from build123d import *

# Parameters (mm, degrees)
EXTRUDE_1_DEPTH     = 6.5
CUT_EXTRUDE_1_REACH = 7
SKETCH_3_R          = 1
CUT_EXTRUDE_2_DEPTH = 3.5
CUT_EXTRUDE_3_DEPTH = 0.5
FILLET_1_R          = 0.2


with BuildPart() as part:
    # 草图1 → 凸台-拉伸1 (new body)
    with BuildSketch(Plane(origin=(0, 0, 0), x_dir=(1, 0, 0), z_dir=(0, 1, 0))):
        with BuildLine():
            Line((-19, 2.5), (19, 2.5))
            ThreePointArc((19, 2.5), (21.5, 0), (19, -2.5))
            Line((19, -2.5), (-19, -2.5))
            ThreePointArc((-19, -2.5), (-21.5, 0), (-19, 2.5))
        make_face()
    extrude(amount=EXTRUDE_1_DEPTH)

    # 草图2 → 切除-拉伸1 (cut, up to next)
    with BuildSketch(Plane.XY.offset(2.5), mode=Mode.PRIVATE) as cut_extrude_1_sk1:
        Polygon((17.468871126, 6.5), (21.5, 4.5), (21.5, 7.438332244), (17.468871126, 7.438332244), align=None)
    cut_extrude_1_tool1 = extrude(cut_extrude_1_sk1.sketch, amount=-CUT_EXTRUDE_1_REACH, mode=Mode.PRIVATE) & part.part
    add(cut_extrude_1_tool1.solids().sort_by_distance((19.83105, 6.383182, 2.5))[0], mode=Mode.SUBTRACT)
    # 草图2 → 切除-拉伸1 (cut, up to next)
    with BuildSketch(Plane.XY.offset(2.5), mode=Mode.PRIVATE) as cut_extrude_1_sk2:
        Polygon((14, 4), (16.5, 0), (16.5, -3.02965668), (-16.5, -3.02965668), (-16.5, 0), (-14, 4), align=None)
    cut_extrude_1_tool2 = extrude(cut_extrude_1_sk2.sketch, amount=-CUT_EXTRUDE_1_REACH, mode=Mode.PRIVATE) & part.part
    add(cut_extrude_1_tool2.solids().sort_by_distance((0, 0.386897, 2.5))[0], mode=Mode.SUBTRACT)
    # 草图2 → 切除-拉伸1 (cut, up to next)
    with BuildSketch(Plane.XY.offset(2.5), mode=Mode.PRIVATE) as cut_extrude_1_sk3:
        Polygon((-21.5, 7.438332244), (-17.468871126, 7.438332244), (-17.468871126, 6.5), (-21.5, 4.5), align=None)
    cut_extrude_1_tool3 = extrude(cut_extrude_1_sk3.sketch, amount=-CUT_EXTRUDE_1_REACH, mode=Mode.PRIVATE) & part.part
    add(cut_extrude_1_tool3.solids().sort_by_distance((-19.83105, 6.383182, 2.5))[0], mode=Mode.SUBTRACT)

    # 草图3 → 切除-拉伸2 (cut)
    with BuildSketch(Plane.XZ):
        with Locations((18.75, 0)):
            Circle(SKETCH_3_R)
        with Locations((-18.75, 0)):
            Circle(SKETCH_3_R)
    extrude(amount=-CUT_EXTRUDE_2_DEPTH, mode=Mode.SUBTRACT)

    # 草图4 → 切除-拉伸3 (cut)
    with BuildSketch(Plane(origin=(0, 6.5, 0), x_dir=(1, 0, 0), z_dir=(0, 1, 0))):
        with BuildLine():
            Line((-9, 1), (9, 1))
            ThreePointArc((9, 1), (10, 0), (9, -1))
            Line((9, -1), (-9, -1))
            ThreePointArc((-9, -1), (-10, 0), (-9, 1))
        make_face()
    extrude(amount=-CUT_EXTRUDE_3_DEPTH, mode=Mode.SUBTRACT)

    # 圆角1
    fillet_1_edges = [part.edges().sort_by_distance(p)[0] for p in [
        (-10, 6, 0),
        (0, 6, -1),
        (10, 6, 0),
        (0, 6, 1),
    ]]
    fillet(fillet_1_edges, radius=FILLET_1_R)


solid = part.part
Geometry: final body of the model. Coordinates: model frame, mm. A direction names the side the tool comes from. Give positions to 0.01 mm unless a question says otherwise; leave off trailing zeros. Write each loop counter-clockwise with the first axis right and the second up, starting at its lowest first coordinate (ties: lowest second). Pieces come first, ordered by that corner, then holes. Notation, with made-up numbers: M 46.25,38 L 69.25,38 A19 ccw 69.25,65 Z; hole C -34.5,5 d11. An arc over 180 degrees is marked long. Answer in a Markdown table with one row per item. Add a question column.
(1) First-contact query: pin 1 (1.5 mm diameter, centred on y = 2, z = 2, fed in from +X); pin 2 (1.5 mm diameter, centred on x = -4.5, y = 1.5, fed in from +Z); pin 3 (0.5 mm diameter, centred on x = -2, z = 0.5, fed in from +Y); pin 4 (2.5 mm diameter, centred on x = 4, z = -0.5, fed in from -Y). Flat tips, straight axial feed; report the tip coordinate or a pass-through.
(2) Ray query, line 1 (Z direction, x = -18.75, y = 2.4); line 2 (X direction, y = 2.25, z = -0.7); line 3 (X direction, y = 2.75, z = 0.25). Return the intervals inside material, ascending.
(3) Section D-D on y = 5. Return loops of the section in (x, z).
(4) Reachability of faces 1 (the flat face through (15.23, 2.03, 0.04)), 2 (the flat face through (0, 6, 0)), 3 (the flat face through (-19, 3.5, 0)) from +Z, -Z, +X, -X, +Y, -Y: full face, straight path, thin tool, end or side. Return the list, or none.
(5) Section C-C on z = 0. Return loops of the section in (x, y), and give its area (3 significant figures).
(6) Section B-B on x = -4. Return loops of the section in (y, z), and give its area (3 significant figures).
(7) Section A-A on y = 2. Return loops of the section in (x, z), and give its area (3 significant figures).
(8) Mould query, pull axis X, two halves, no side actions, for faces 4 (the flat face through (-15.27, 1.97, 0.04)), 5 (the cylindrical face through (21.5, 2.2, -0.1)), 6 (the cylindrical face through (-21.5, 2.2, 0.1)), 7 (the flat face through (0, 4, 0)). Classes: +X half, -X half, draft (parallel to the pull), parting line (faces both ways), or undercut.
Result set:
| question | item | result |
|---|---|---|
| 1 | pin 1 | stops at x = 21.17 |
| 1 | pin 2 | passes through |
| 1 | pin 3 | stops at y = 6 |
| 1 | pin 4 | stops at y = 4 |
| 2 | line 1 | z = -2.5 to -1, 1 to 2.5 |
| 2 | line 2 | x = -21.4 to -19.46, -18.04 to -15.09, 15.09 to 18.04, 19.46 to 21.4 |
| 2 | line 3 | x = -21.49 to -19.72, -17.78 to -14.78, 14.78 to 17.78, 19.72 to 21.49 |
| 3 | outline | M -20.49,-2.01 A2.5 ccw -19,-2.5 L 19,-2.5 A2.5 ccw 20.49,-2.01 L 20.49,2.01 A2.5 ccw 19,2.5 L -19,2.5 A2.5 ccw -20.49,2.01 Z |
| 4 | face 1 | +Z, -Z, -Y |
| 4 | face 2 | +Y |
| 4 | face 3 | -Y |
| 5 | outline | M -21.5,0 L -19.75,0 L -19.75,3.5 L -17.75,3.5 L -17.75,0 L -16.5,0 L -14,4 L 14,4 L 16.5,0 L 17.75,0 L 17.75,3.5 L 19.75,3.5 L 19.75,0 L 21.5,0 L 21.5,4.5 L 17.47,6.5 L 10,6.5 L 10,6.2 A0.2 cw 9.8,6 L -9.8,6 A0.2 cw -10,6.2 L -10,6.5 L -17.47,6.5 L -21.5,4.5 Z |
| 5 | area | 125 mm^2 |
| 6 | outline | M 4,-2.5 L 6.5,-2.5 L 6.5,-1 L 6.2,-1 A0.2 cw 6,-0.8 L 6,0.8 A0.2 cw 6.2,1 L 6.5,1 L 6.5,2.5 L 4,2.5 Z |
| 6 | area | 11.5 mm^2 |
| 7 | outline | M -19,-2.5 L -15.25,-2.5 L -15.25,2.5 L -19,2.5 A2.5 ccw Z; M 15.25,-2.5 L 19,-2.5 A2.5 ccw 19,2.5 L 15.25,2.5 Z; hole C -18.75,0 d2; hole C 18.75,0 d2 |
| 7 | area | 50.9 mm^2 |
| 8 | face 4 | undercut |
| 8 | face 5 | +X half |
| 8 | face 6 | -X half |
| 8 | face 7 | undercut |
